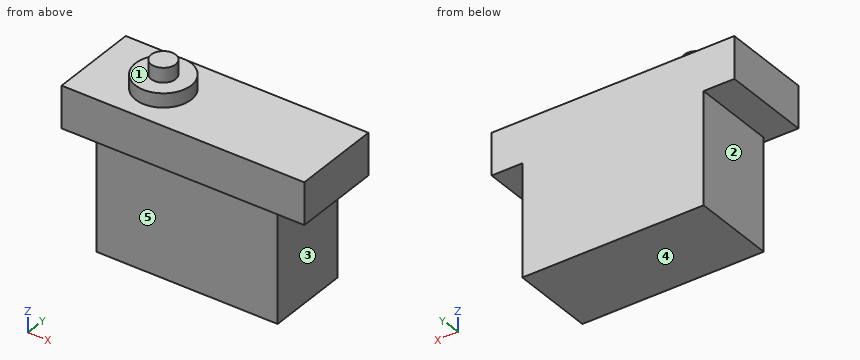
```python
from build123d import *

# Parameters (mm, degrees)
F0_W     = 41.275
F0_H     = 19.05
F1_DEPTH = 25.4
F2_W     = 55.245
F2_H     = 20.32
F3_DEPTH = 9.525
F4_R     = 6.35
F5_DEPTH = 3.175
F6_R     = 2.794
F7_DEPTH = 3.302


with BuildPart() as f1:
    # F0 (on Top) → F1 (new body)
    with BuildSketch(Plane.XY):
        with Locations((-16.2392864004, 7.7934292579)):
            Rectangle(F0_W, F0_H)
    extrude(amount=F1_DEPTH)

    # F2 (on face) → F3 (join)
    with BuildSketch(Plane.XY.offset(25.4)):
        with Locations((-16.2392864004, 7.1584292579)):
            Rectangle(F2_W, F2_H)
    extrude(amount=F3_DEPTH)

    # F4 (on face) → F5 (join)
    with BuildSketch(Plane.XY.offset(34.925)):
        with Locations((-27.9867864004, 7.1584292579)):
            Circle(F4_R)
    extrude(amount=F5_DEPTH)

    # F6 (on face) → F7 (join)
    with BuildSketch(Plane.XY.offset(38.1)):
        with Locations((-27.9867864004, 7.1584292579)):
            Circle(F6_R)
    extrude(amount=F7_DEPTH)


solid = f1.part
```
Verification items for the finished model (mm, model axes). Face numbers are marked on the shaded views. A direction names the side the tool comes from. Round coordinates to 2 decimals unless told otherwise and drop trailing zeros. Write each loop counter-clockwise with the first axis right and the second up, starting at its lowest first coordinate (ties: lowest second). Pieces come first, ordered by that corner, then holes. Notation, with made-up numbers: (62, 67) - (66, 67) arc R18 cw to (66, 102) - close; hole circle Ø9 at (42.25, -22.5). An arc over 180 degrees is marked (long way). Answer as a JSON object with one key per item and string values. Group by question number.
Q1. Section check D-D, the plane x = -31.5. Enter the section's corners in (y, z) (3 decimals), plus the area to 3 significant figures.
Q2. Section check B-B, the plane y = 16.25. Enter the section's corners in (x, z) (3 decimals), plus the area to 3 significant figures.
Q3. Go/stop test with flat-tipped pins: pin 1 Ø9.5 at (y, z) = (9, 10) entering from -X; pin 2 Ø1.5 at (x, y) = (-24.5, 0) entering from +Z (3 decimals); pin 3 Ø5.5 at (y, z) = (9.5, 14) entering from +X; pin 4 Ø6 at (x, y) = (-19.5, 3) entering from -Z. Record where each tip stops, or that it passes through.
Q4. Section check C-C, the plane z = 21. Enter the section's corners in (x, y), plus the area to 3 significant figures.
Q5. Section check A-A, the plane x = 1. Enter the section's corners in (y, z) (3 decimals).
Q6. Tool access check on the marked faces 1, 2, 3, 4 and 5. Record the directions out of +Z, -Z, +X, -X, +Y, -Y that give a thin tool (end or side, any length) a straight path to the whole face; none if there is none.
Q7. Thickness scan on line 1 (Y direction, x = -21, z = 14); line 2 (Z direction, x = 4, y = 7.5) (3 decimals); line 3 (X direction, y = 12.25, z = 20). Record the ranges inside material, lowest first.
Found:
{
 "1": {"outline": "(-3.002, 25.4) - (-1.732, 25.4) - (-1.732, 0) - (17.318, 0) - (17.318, 34.925) - (12.448, 34.925) - (12.448, 38.1) - (1.869, 38.1) - (1.869, 34.925) - (-3.002, 34.925) - close", "area": "711 mm^2"},
 "2": {"outline": "(-43.862, 25.4) - (-36.877, 25.4) - (-36.877, 0) - (4.398, 0) - (4.398, 25.4) - (11.383, 25.4) - (11.383, 34.925) - (-43.862, 34.925) - close", "area": "1,570 mm^2"},
 "3": {"pin 1": "stops at x = -36.88", "pin 2": "stops at z = 34.925", "pin 3": "stops at x = 4.4", "pin 4": "stops at z = 0"},
 "4": {"outline": "(-36.88, -1.73) - (4.4, -1.73) - (4.4, 17.32) - (-36.88, 17.32) - close", "area": "786 mm^2"},
 "5": {"outline": "(-3.002, 25.4) - (-1.732, 25.4) - (-1.732, 0) - (17.318, 0) - (17.318, 34.925) - (-3.002, 34.925) - close"},
 "6": {"face 1": "+Z", "face 2": "-Z, -X, +Y, -Y", "face 3": "-Z, +X, +Y, -Y", "face 4": "-Z, +X, -X, +Y, -Y", "face 5": "-Z, +X, -X, -Y"},
 "7": {"line 1": "y = -1.73 to 17.32", "line 2": "z = 0 to 34.925", "line 3": "x = -36.88 to 4.4"}
}
